Autodesk Inventor part; units mm, degrees
ref_plane "YZ Plane" through (0, 0, 0) normal (1, 0, 0) x (0, 1, 0)
ref_plane "XZ Plane" through (0, 0, 0) normal (0, 1, 0) x (-1, 0, 0)
ref_plane "XY Plane" through (0, 0, 0) normal (0, 0, 1) x (1, 0, 0)
sketch "Sketch1" plane through (0, 0, 0) normal (0, 1, 0) x (-1, 0, 0)
  line L0 (-101.6, -101.6) -> (101.6, -101.6)
  line L1 (101.6, -101.6) -> (101.6, 101.6)
  line L2 (101.6, 101.6) -> (-101.6, 101.6)
  line L3 (-101.6, 101.6) -> (-101.6, -101.6)
  line L4 (-101.6, -101.6) -> (101.6, 101.6) construction
  line L5 (101.6, -101.6) -> (-101.6, 101.6) construction
  point P0 (0, 0)
  dimension "d0" = 203.2
  dimension "d1" = 203.2
extrude "Extrusion1" add sketch "Sketch1" along normal mid plane 304.8
sketch "Sketch2" plane through (101.6, -152.4, -101.6) normal (1, 0, 0) x (0, 0, -1)
  line L0 (0, 304.8) -> (-203.2, 304.8)
  line L1 (-101.6, 304.8) -> (-203.2, 152.4)
  line L2 (-203.2, 0) -> (-203.2, 304.8)
  line L3 (-203.2, 152.4) -> (-101.6, 0)
  line L4 (0, 0) -> (-203.2, 0)
  line L5 (-101.6, 0) -> (0, 152.4)
  line L6 (0, 0) -> (0, 304.8)
  line L7 (-101.6, 304.8) -> (0, 152.4)
  point P0 (-101.6, 152.4)
extrude "Extrusion2" cut sketch "Sketch2" against normal blind 304.8 contours L6 L7 L0 | L1 L2 L0 | L6 L4 L5 | L3 L4 L2
sketch "Sketch3" plane through (0, 0, 0) normal (0, 0, 1) x (1, 0, 0)
  line L0 (-101.6, 152.4) -> (101.6, 152.4)
  line L1 (0, 152.4) -> (-101.6, 0)
  line L2 (-101.6, 0) -> (0, -152.4)
  line L3 (-101.6, -152.4) -> (101.6, -152.4)
  line L4 (101.6, 0) -> (101.6, -152.4)
  line L5 (101.6, 0) -> (0, 152.4)
  line L6 (101.6, 0) -> (0, -152.4)
  line L7 (-101.6, 0) -> (-101.6, 152.4)
  line L8 (-101.6, 0) -> (101.6, 0)
  line L9 (101.6, 152.4) -> (101.6, 0)
  line L10 (-101.6, 152.4) -> (101.6, 152.4)
  line L11 (-101.6, -152.4) -> (-101.6, 0)
  line L12 (-101.6, -152.4) -> (101.6, -152.4)
  line L13 (101.6, 0) -> (101.6, -152.4)
  line L14 (-101.6, 0) -> (101.6, 0)
  point P0 (0, 0)
extrude "Extrusion3" cut sketch "Sketch3" along normal through all both and the other way through all contours L0 L1 L7 | L0 L9 L5 | L2 L3 L11 | L4 L3 L6
properties part number "Dice, Simplified" material "PVC-Piping"
Input: part model. Units: mm. Frame: model coordinates. Round coordinates to 2 decimals unless told otherwise and drop trailing zeros. Write each loop counter-clockwise with the first axis right and the second up, starting at its lowest first coordinate (ties: lowest second). Pieces come first, ordered by that corner, then holes.
1) Cut plane D-D (y = 10.5). Return the cut outline in (x, z), then the cut area to 3 significant figures.
2) Cut plane B-B (y = -69). Return the cut outline in (x, z).
3) Cut plane C-C (x = 31.5). Return the cut outline in (y, z).
4) Cut plane A-A (z = 76). Return the cut outline in (x, y).
5) Ray query, L1, parallel to Z at x = 62, y = 47; L2, parallel to Z at x = -13, y = 11; L3, parallel to Y at x = 22, z = 29. Return the intervals inside material, ascending.
6) Contact query for flat-ended pins moving along their axis: P1, Ø8, axis at x = 17.5, z = 13.5, coming from the +Y side; P2, Ø10, axis at x = -12, y = -11, coming from the -Z side; P3, Ø5, axis at x = -58.5, y = -12.5, coming from the -Z side. Output: stop coordinate, or through.
Geometry says:
1. outline: (-94.6, -94.6) - (94.6, -94.6) - (94.6, 94.6) - (-94.6, 94.6) - close
1. area: 35,800 mm2
2. outline: (-55.6, -55.6) - (55.6, -55.6) - (55.6, 55.6) - (-55.6, 55.6) - close
3. outline: (-105.15, -31.5) - (0, -101.6) - (105.15, -31.5) - (105.15, 31.5) - (0, 101.6) - (-105.15, 31.5) - close
4. outline: (-101.6, 0) - (-76, -38.4) - (76, -38.4) - (101.6, 0) - (76, 38.4) - (-76, 38.4) - close
5. L1: z = -70.27 to 70.27
5. L2: z = -94.27 to 94.27
5. L3: y = -108.9 to 108.9
6. P1: stops at y = 132.15
6. P2: stops at z = -97.6
6. P3: stops at z = -94.93
